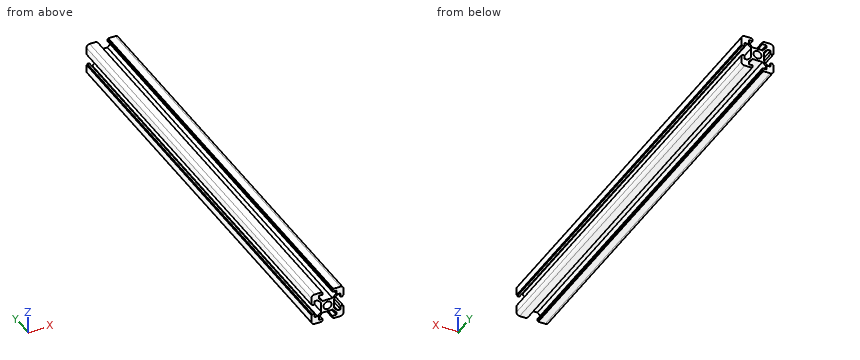
```python
from build123d import *

# Parameters (mm, degrees)
SKETCH_1_R      = 2.5
EXTRUDE_1_DEPTH = 270


with BuildPart() as part:
    # 草图1 → 凸台-拉伸1 (new body)
    with BuildSketch(Plane(origin=(0, 0, 0), x_dir=(1, 0, 0), z_dir=(0, 1, 0))):
        with BuildLine():
            Line((-3.948528137, -3.1), (-6.298528137, -5.45))
            Line((-6.298528137, -5.45), (-8.2, -5.45))
            Line((-8.2, -5.45), (-8.2, -3.1))
            Line((-8.2, -3.1), (-9.5, -3.1))
            Line((-9.5, -3.1), (-9.5, -3.6))
            Line((-9.5, -3.6), (-10, -3.6))
            Line((-10, -3.6), (-10, -8))
            ThreePointArc((-10, -8), (-9.414213562, -9.414213562), (-8, -10))
            Line((-8, -10), (-3.6, -10))
            Line((-3.6, -10), (-3.6, -9.5))
            Line((-3.6, -9.5), (-3.1, -9.5))
            Line((-3.1, -9.5), (-3.1, -8.2))
            Line((-3.1, -8.2), (-5.45, -8.2))
            Line((-5.45, -8.2), (-5.45, -6.298528137))
            Line((-5.45, -6.298528137), (-3.1, -3.948528137))
            Line((-3.1, -3.948528137), (0, -3.948528137))
            Line((0, -3.948528137), (3.1, -3.948528137))
            Line((3.1, -3.948528137), (5.45, -6.298528137))
            Line((5.45, -6.298528137), (5.45, -8.2))
            Line((5.45, -8.2), (3.1, -8.2))
            Line((3.1, -8.2), (3.1, -9.5))
            Line((3.1, -9.5), (3.6, -9.5))
            Line((3.6, -9.5), (3.6, -10))
            Line((3.6, -10), (8, -10))
            ThreePointArc((8, -10), (9.414213562, -9.414213562), (10, -8))
            Line((10, -8), (10, -3.6))
            Line((10, -3.6), (9.5, -3.6))
            Line((9.5, -3.6), (9.5, -3.1))
            Line((9.5, -3.1), (8.2, -3.1))
            Line((8.2, -3.1), (8.2, -5.45))
            Line((8.2, -5.45), (6.298528137, -5.45))
            Line((6.298528137, -5.45), (3.948528137, -3.1))
            Line((3.948528137, -3.1), (3.948528137, 0))
            Line((3.948528137, 0), (3.948528137, 3.1))
            Line((3.948528137, 3.1), (6.298528137, 5.45))
            Line((6.298528137, 5.45), (8.2, 5.45))
            Line((8.2, 5.45), (8.2, 3.1))
            Line((8.2, 3.1), (9.5, 3.1))
            Line((9.5, 3.1), (9.5, 3.6))
            Line((9.5, 3.6), (10, 3.6))
            Line((10, 3.6), (10, 8))
            ThreePointArc((10, 8), (9.414213562, 9.414213562), (8, 10))
            Line((8, 10), (3.6, 10))
            Line((3.6, 10), (3.6, 9.5))
            Line((3.6, 9.5), (3.1, 9.5))
            Line((3.1, 9.5), (3.1, 8.2))
            Line((3.1, 8.2), (5.45, 8.2))
            Line((5.45, 8.2), (5.45, 6.298528137))
            Line((5.45, 6.298528137), (3.1, 3.948528137))
            Line((3.1, 3.948528137), (0, 3.948528137))
            Line((0, 3.948528137), (-3.1, 3.948528137))
            Line((-3.1, 3.948528137), (-5.45, 6.298528137))
            Line((-5.45, 6.298528137), (-5.45, 8.2))
            Line((-5.45, 8.2), (-3.1, 8.2))
            Line((-3.1, 8.2), (-3.1, 9.5))
            Line((-3.1, 9.5), (-3.6, 9.5))
            Line((-3.6, 9.5), (-3.6, 10))
            Line((-3.6, 10), (-8, 10))
            ThreePointArc((-8, 10), (-9.414213562, 9.414213562), (-10, 8))
            Line((-10, 8), (-10, 3.6))
            Line((-10, 3.6), (-9.5, 3.6))
            Line((-9.5, 3.6), (-9.5, 3.1))
            Line((-9.5, 3.1), (-8.2, 3.1))
            Line((-8.2, 3.1), (-8.2, 5.45))
            Line((-8.2, 5.45), (-6.298528137, 5.45))
            Line((-6.298528137, 5.45), (-3.948528137, 3.1))
            Line((-3.948528137, 3.1), (-3.948528137, 0))
            Line((-3.948528137, 0), (-3.948528137, -3.1))
        make_face()
        with Locations(Location((0, 0, 0), (0, 0, 270))):
            Circle(SKETCH_1_R, mode=Mode.SUBTRACT)
    extrude(amount=EXTRUDE_1_DEPTH)


solid = part.part
```
Geometry: final body of the model. Coordinates: model frame, mm. Round coordinates to 2 decimals unless told otherwise and drop trailing zeros. Loops run counter-clockwise (first coordinate to the right, second up) from the corner with the lowest first, then second, coordinate; pieces in that order, holes last.
Item 1: Section A-A, the plane x = 0. Output: boundary loops of the cut face in (y, z), plus the area to 3 significant figures.
Checked values:
outline: (0, -3.95) - (270, -3.95) - (270, -2.5) - (0, -2.5) - close; (0, 2.5) - (270, 2.5) - (270, 3.95) - (0, 3.95) - close
area: 782 mm2
Item 2: Contact query for flat-ended pins moving along their axis: P1, Ø1.4, axis at y = 201.5, z = -9, coming from the -X side; P2, Ø1.4, axis at x = 9, y = 86, coming from the +Z side; P3, Ø0.7, axis at y = 116, z = -9, coming from the +X side. Output: stop coordinate, or through.
Checked values:
P1: stops at x = -9.98
P2: stops at z = 9.98
P3: stops at x = 9.89
Item 3: Line query: L1, parallel to X at y = 151, z = -7.25; L2, parallel to X at y = 162, z = -3.25; L3, parallel to X at y = 216.5, z = 0. Output: solid intervals per line, ascending.
Checked values:
L1: x = -10 to -5.45, 5.45 to 10
L2: x = -9.5 to -8.2, -4.1 to 4.1, 8.2 to 9.5
L3: x = -3.95 to -2.5, 2.5 to 3.95
